Check sheet for the modelled part. Datum: model origin and axes. Units: mm. A direction names the side the tool comes from. Coordinates: 2 decimals unless noted, no trailing zeros. Write each loop counter-clockwise with the first axis right and the second up, starting at its lowest first coordinate (ties: lowest second). Pieces come first, ordered by that corner, then holes. Notation, with made-up numbers: (24, -17.75) -> (64, -17.75) arc R26 cw to (64, -3.75) -> close; hole circle Ø6 at (79.5, -2.5). An arc over 180 degrees is marked (long way). Put each result on its own line as item: value.
Solid Edge part; units mm, degrees
sketch "Sketch1" plane through (0, 0, 0) normal (0, 0, 1) x (1, 0, 0)
  line L0 (-43.5, -38) -> (43.5, -38)
  line L1 (43.5, -38) -> (43.5, 38)
  line L2 (43.5, 38) -> (-43.5, 38)
  line L3 (-43.5, 38) -> (-43.5, -38)
extrude "Protrusion1" add sketch "Sketch1" against normal blind 15
sketch "Sketch2" plane through (0, 0, 0) normal (0, 0, 1) x (1, 0, 0)
  line L0 (-43.5, 38) -> (-11, 38)
  line L1 (-11, 38) -> (-11, 22)
  line L2 (-11, 22) -> (-43.5, 22)
  line L3 (-43.5, 22) -> (-43.5, 38)
  line L4 (43.5, 38) -> (11, 38)
  line L5 (11, 38) -> (11, 22)
  line L6 (11, 22) -> (43.5, 22)
  line L7 (43.5, 22) -> (43.5, 38)
extrude "ExtrudedCutout_1" cut sketch "Sketch2" against normal blind 15
sketch "Sketch3" plane through (0, 0, 0) normal (0, 0, 1) x (1, 0, 0)
  line L0 (-43.5, 22) -> (-4.5, 22)
  line L1 (-4.5, 22) -> (-4.5, 17)
  line L2 (-4.5, 17) -> (-43.5, 17)
  line L3 (-43.5, 17) -> (-43.5, 22)
  line L4 (43.5, 22) -> (4.5, 22)
  line L5 (4.5, 22) -> (4.5, 17)
  line L6 (4.5, 17) -> (43.5, 17)
  line L7 (43.5, 17) -> (43.5, 22)
extrude "ExtrudedCutout_2" cut sketch "Sketch3" against normal blind 15
sketch "Sketch4" plane through (0, 0, 0) normal (0, 0, 1) x (1, 0, 0)
  line L0 (-43.5, 17) -> (-14.5, 17)
  line L1 (-14.5, 17) -> (-14.5, 9)
  line L2 (-14.5, 9) -> (-43.5, 9)
  line L3 (-43.5, 9) -> (-43.5, 17)
  line L4 (43.5, 17) -> (14.5, 17)
  line L5 (14.5, 17) -> (14.5, 9)
  line L6 (14.5, 9) -> (43.5, 9)
  line L7 (43.5, 9) -> (43.5, 17)
extrude "ExtrudedCutout_3" cut sketch "Sketch4" against normal blind 15
sketch "Sketch5" plane through (0, 0, 0) normal (0, 0, 1) x (1, 0, 0)
  line L0 (-23.5, 9) -> (-43.5, -38)
  line L1 (-43.5, -38) -> (-43.5, 9)
  line L2 (-43.5, 9) -> (-23.5, 9)
  line L3 (23.5, 9) -> (43.5, -38)
  line L4 (43.5, -38) -> (43.5, 9)
  line L5 (43.5, 9) -> (23.5, 9)
extrude "ExtrudedCutout_4" cut sketch "Sketch5" against normal blind 15
fillet "Round_1" radius 3 8 edges at (23.5, 9, -7.5) (11, 22, -7.5) (11, 38, -7.5) (14.5, 17, -7.5) (-11, 38, -7.5) (-11, 22, -7.5) (-14.5, 17, -7.5) (-23.5, 9, -7.5)
fillet "Round_2" radius 2 2 edges at (43.5, -38, -7.5) (-43.5, -38, -7.5)
sketch "Sketch6" plane through (0, 0, 0) normal (0, 0, 1) x (1, 0, 0)
  circle A0 centre (0, 31.0011) radius 3.15
extrude "ExtrudedCutout_5" cut sketch "Sketch6" against normal blind 15
Q1. Cross-section at C-C (x = 34.5). Record the cut outline in (y, z), plus the area to 3 significant figures.
Recorded:
outline: (-38, -15) -> (-16.85, -15) -> (-16.85, 0) -> (-38, 0) -> close
area: 317 mm2
Q2. Material ranges on line 1 along Y through (x, z) = (0, -5.75); line 2 along Y through (x, z) = (9, -4); line 3 along X through (y, z) = (11, -1.75), recorded low to high.
Recorded:
line 1: y = -38 to 27.85, 34.15 to 38
line 2: y = -38 to 17, 22.17 to 37.83
line 3: x = -14.5 to 14.5
Q3. Depth check by flat-ended pin: P1, Ø3.5, axis at x = 18, z = -8.5, coming from the +Y side; P2, Ø2.5, axis at y = 11.5, z = -6, coming from the +X side; P3, Ø8, axis at y = 31.5, z = -4.5, coming from the +X side; P4, Ø5, axis at x = 0, y = 31, coming from the -Z side. Enter the tip coordinate at first touch or a pass-through.
Recorded:
P1: stops at y = 9
P2: stops at x = 14.5
P3: stops at x = 11
P4: passes through
Q4. Cross-section at D-D (y = -16). Record the cut outline in (x, z), plus the area to 3 significant figures.
Recorded:
outline: (-34.14, -15) -> (34.14, -15) -> (34.14, 0) -> (-34.14, 0) -> close
area: 1,020 mm2
Q5. Mould release check, pull along Y, two halves, no side actions. Record for faces 1 (the cylindrical face through (42.16, -37.08, -7.6)), 2 (the flat face through (-1, -38, -7)), 3 (the flat face through (6, 22, -7)), 4 (the flat face through (14.5, 12, -7)): released by +Y, released by -Y, zero draft, split by the parting line, or undercut.
Recorded:
face 1: split by the parting line
face 2: released by -Y
face 3: undercut
face 4: zero draft
Q6. Cross-section at B-B (z = -13.5). Record the cut outline in (x, y), plus the area to 3 significant figures.
Recorded:
outline: (-42.32, -35.22) arc R2 ccw to (-40.48, -38) -> (40.48, -38) arc R2 ccw to (42.32, -35.22) -> (24.28, 7.17) arc R3 ccw to (21.52, 9) -> (14.5, 9) -> (14.5, 14) arc R3 ccw to (11.5, 17) -> (4.5, 17) -> (4.5, 22) -> (8, 22) arc R3 ccw to (11, 25) -> (11, 35) arc R3 ccw to (8, 38) -> (-8, 38) arc R3 ccw to (-11, 35) -> (-11, 25) arc R3 ccw to (-8, 22) -> (-4.5, 22) -> (-4.5, 17) -> (-11.5, 17) arc R3 ccw to (-14.5, 14) -> (-14.5, 9) -> (-21.52, 9) arc R3 ccw to (-24.28, 7.17) -> close; hole circle Ø6.3 at (0, 31)
area: 3,730 mm2
Q7. Tool access check on faces 5 (the flat face through (-1, -8, 0)), 6 (the flat face through (18, 9, -7)), 7 (the flat face through (-4.5, 20, -7)), 8 (the flat face through (-11, 30, -7)), 9 (the cylindrical face through (-0.683, 27.926, -7.395)). Record the directions out of +Z, -Z, +X, -X, +Y, -Y that give a thin tool (end or side, any length) a straight path to the whole face; none if there is none.
Recorded:
face 5: +Z, +X, -X, +Y, -Y
face 6: +Z, -Z, +X, +Y
face 7: +Z, -Z, -X
face 8: +Z, -Z, -X, +Y
face 9: +Z, -Z
Q8. Cross-section at A-A (x = 0). Record the cut outline in (y, z).
Recorded:
outline: (-38, -15) -> (27.85, -15) -> (27.85, 0) -> (-38, 0) -> close; (34.15, -15) -> (38, -15) -> (38, 0) -> (34.15, 0) -> close
